For this review, take the finished solid that the model builds, in its own axes (mm). A direction names the side the tool comes from. Round coordinates to 2 decimals unless told otherwise and drop trailing zeros. Write each loop counter-clockwise with the first axis right and the second up, starting at its lowest first coordinate (ties: lowest second). Pieces come first, ordered by that corner, then holes. Notation, with made-up numbers: (10.5, 54.5) - (34.5, 54.5) arc R5 cw to (34.5, 62.5) - close; hole circle Ø3 at (26.25, 58). An arc over 180 degrees is marked (long way). Answer in a Markdown table with one row per item. Add a question column.
from build123d import *

# Parameters (mm, degrees)
F1_DEPTH = 3.81
F3_DEPTH = 12.7
F4_SIZE  = 1.27


with BuildPart() as f1:
    # F0 (on Front) → F1 (new body)
    with BuildSketch(Plane.XZ):
        with BuildLine():
            ThreePointArc((25.4, 10.795), (23.912102, 14.387102), (20.32, 15.875))
            Line((20.32, 15.875), (9.525, 15.875))
            ThreePointArc((9.525, 15.875), (0, 6.35), (-9.525, 15.875))
            Line((-9.525, 15.875), (-20.32, 15.875))
            ThreePointArc((-20.32, 15.875), (-23.912102, 14.387102), (-25.4, 10.795))
            Line((-25.4, 10.795), (-25.4, -15.875))
            Line((-25.4, -15.875), (25.4, -15.875))
            Line((25.4, -15.875), (25.4, 10.795))
        make_face()
    extrude(amount=F1_DEPTH)

    # F2 (on face) → F3 (join)
    with BuildSketch(Plane.XZ.offset(3.81)):
        with BuildLine():
            ThreePointArc((9.525, 15.875), (0, 6.35), (-9.525, 15.875))
            Line((-9.525, 15.875), (-12.065, 15.875))
            Line((-12.065, 15.875), (-12.065, 5.08))
            ThreePointArc((-12.065, 5.08), (-13.552898, 1.487898), (-17.145, 0))
            Line((-17.145, 0), (-20.32, 0))
            Line((-20.32, 0), (-20.32, -15.875))
            Line((-20.32, -15.875), (-15.24, -15.875))
            Line((-15.24, -15.875), (-15.24, -6.985))
            Line((-15.24, -6.985), (0, -6.985))
            Line((0, -6.985), (15.24, -6.985))
            Line((15.24, -6.985), (15.24, -15.875))
            Line((15.24, -15.875), (20.32, -15.875))
            Line((20.32, -15.875), (20.32, 0))
            Line((20.32, 0), (17.145, 0))
            ThreePointArc((17.145, 0), (13.552898, 1.487898), (12.065, 5.08))
            Line((12.065, 5.08), (12.065, 15.875))
            Line((12.065, 15.875), (9.525, 15.875))
        make_face()
    extrude(amount=F3_DEPTH)

    # F4
    f4_edges = [f1.edges().sort_by_distance(p)[0] for p in [
        (0, -16.51, 6.35),
        (-15.24, -16.51, -11.43),
        (0, -16.51, -6.985),
        (15.24, -16.51, -11.43),
    ]]
    chamfer(f4_edges, length=F4_SIZE)


solid = f1.part
Q1. Add section D-D on y = -8. State the section outline as (x, z) points (3 decimals), then the cut area to 3 significant figures.
Q2. Tool access review of faces 1 (the face through (16, -16, -11)), 2 (the face through (-20.32, -10, -8)), 3 (the face through (20.32, -10, -8)): name each direction out of +Z, -Z, +X, -X, +Y, -Y from which nothing blocks a thin tool from reaching the whole face with its end or side.
Q3. Insertion check: pin 1 Ø6 at (y, z) = (-13, 10.5) entering from +X (3 decimals); pin 2 Ø2 at (y, z) = (-8, -6) entering from -X; pin 3 Ø10.5 at (x, z) = (21.5, 5.5) entering from -Y. Each pin has a flat end and moves straight along its axis. Give the tip position at first contact, or say it passes through.
Q4. Add section A-A on y = -2.5. State the section outline as (x, z) points (3 decimals).
Q5. Draft analysis for pull direction X (two halves, no side actions). For faces 4 (the face through (15.24, -9, -11)), 5 (the face through (0.21, -15.46, 6.13)), 6 (the face through (0, -16.51, -2)), 7 (the face through (12.065, -10, 10)), state which applies: released by +X, released by -X, zero draft, split by the parting line, or undercut.
Q6. Add section C-C on x = 0. State the section outline as (y, z) points (3 decimals), then the cut area to 3 significant figures.
Q7. Add section B-B on z = -13.5. State the section outline as (x, y) points, then the cut area to 3 significant figures.
Q8. To check wall thickness, follow probe 1 along X at (y, z) = (-5, -10.5); probe 2 along Z at (x, y) = (20, -15.5) (3 decimals); probe 3 along X at (y, z) = (-4.75, 14.5) (3 decimals). State the ranges of each line that lie inside material, in increasing order.
Answer sheet:
| question | item | result |
|---|---|---|
| 1 | outline | (-20.32, -15.875) - (-15.24, -15.875) - (-15.24, -6.985) - (15.24, -6.985) - (15.24, -15.875) - (20.32, -15.875) - (20.32, 0) - (17.145, 0) arc R5.08 cw to (12.065, 5.08) - (12.065, 15.875) - (9.525, 15.875) arc R9.525 cw to (-9.525, 15.875) - (-12.065, 15.875) - (-12.065, 5.08) arc R5.08 cw to (-17.145, 0) - (-20.32, 0) - close |
| 1 | area | 626 mm² |
| 2 | face 1 | -Z, -Y |
| 2 | face 2 | +Z, -Z, -X, -Y |
| 2 | face 3 | +Z, -Z, +X, -Y |
| 3 | pin 1 | stops at x = 12.065 |
| 3 | pin 2 | stops at x = -20.32 |
| 3 | pin 3 | stops at y = -3.81 |
| 4 | outline | (-25.4, -15.875) - (25.4, -15.875) - (25.4, 10.795) arc R5.08 ccw to (20.32, 15.875) - (9.525, 15.875) arc R9.525 cw to (-9.525, 15.875) - (-20.32, 15.875) arc R5.08 ccw to (-25.4, 10.795) - close |
| 5 | face 4 | undercut |
| 5 | face 5 | undercut |
| 5 | face 6 | zero draft |
| 5 | face 7 | released by +X |
| 6 | outline | (-16.51, -5.715) - (-15.24, -6.985) - (-3.81, -6.985) - (-3.81, -15.875) - (0, -15.875) - (0, 6.35) - (-15.24, 6.35) - (-16.51, 5.08) - close |
| 6 | area | 252 mm² |
| 7 | outline | (-25.4, -3.81) - (-20.32, -3.81) - (-20.32, -16.51) - (-16.51, -16.51) - (-15.24, -15.24) - (-15.24, -3.81) - (15.24, -3.81) - (15.24, -15.24) - (16.51, -16.51) - (20.32, -16.51) - (20.32, -3.81) - (25.4, -3.81) - (25.4, 0) - (-25.4, 0) - close |
| 7 | area | 321 mm² |
| 8 | probe 1 | x = -20.32 to -15.24, 15.24 to 20.32 |
| 8 | probe 2 | z = -15.875 to 0 |
| 8 | probe 3 | x = -12.065 to -9.425, 9.425 to 12.065 |
